Geometry: final body of the model. Coordinates: model frame, mm. A direction names the side the tool comes from. Round coordinates to 2 decimals unless told otherwise and drop trailing zeros. Loops run counter-clockwise (first coordinate to the right, second up) from the corner with the lowest first, then second, coordinate; pieces in that order, holes last. Notation, with made-up numbers: M 13.25,15.25 L 33.25,15.25 A18 ccw 33.25,29.25 Z; hole C 52,-18.5 d7. An arc over 180 degrees is marked long. Return JSON: item names as keys, results as strings.
Autodesk Fusion 360 part; units mm, degrees
sketch "Sketch1" plane through (0, 0, 0) normal (0, 0, 1) x (1, 0, 0) in component "Headpost"
  line L0 (7.5, -5) -> (-7.5, -5)
  line L1 (-7.5, -5) -> (-7.5, 5)
  line L2 (-7.5, 5) -> (7.5, 5)
  line L3 (7.5, 5) -> (7.5, -5)
  line L4 (7.5, -5) -> (-7.5, 5) construction
  line L5 (-7.5, -5) -> (7.5, 5) construction
  dimension "d1" = 15
  dimension "d2" = 10
extrude "Extrude1" add sketch "Sketch1" along normal blind 10 in component "Headpost"
sketch "Sketch2" plane through (0, 0, 10) normal (0, 0, 1) x (-1, 0, 0) in component "Headpost"
  line L0 (-7.5, -5) -> (7.5, -5)
  line L1 (7.5, -5) -> (7.5, 5)
  line L2 (7.5, 5) -> (-7.5, 5)
  line L3 (-7.5, 5) -> (-7.5, -5)
  line L4 (6, 3.5) -> (-6, 3.5)
  line L5 (-6, 3.5) -> (-6, -3.5)
  line L6 (-6, -3.5) -> (6, -3.5)
  line L7 (6, -3.5) -> (6, 3.5)
  dimension "d5" = -1.5
extrude "Extrude2" cut sketch "Sketch2" against normal blind 15 contours L4 L5 L6 L7 in component "Headpost"
sketch "Sketch3" plane through (-7.5, 0, 0) normal (-1, 0, 0) x (0, -1, 0) in component "Headpost"
  line L0 (-5, 0) -> (5, 0)
  line L1 (5, 0) -> (5, 10)
  line L2 (5, 10) -> (-5, 10)
  line L3 (-5, 10) -> (-5, 0)
  line L4 (-5, 10) -> (5, 10)
  line L5 (5, 10) -> (5, 8)
  line L6 (5, 8) -> (-5, 8)
  line L7 (-5, 8) -> (-5, 10)
  dimension "d8" = 10
  dimension "d9" = 2
extrude "Extrude3" add sketch "Sketch3" along normal blind 7.5 contours L1 L2 L3 L4 L5 L6 L7 in component "Headpost"
sketch "Sketch4" plane through (7.5, 0, 0) normal (1, 0, 0) x (0, 1, 0) in component "Headpost"
  line L0 (-5, 0) -> (5, 0)
  line L1 (5, 0) -> (5, 10)
  line L2 (5, 10) -> (-5, 10)
  line L3 (-5, 10) -> (-5, 0)
  line L4 (-5, 10) -> (5, 10)
  line L5 (5, 10) -> (5, 8)
  line L6 (5, 8) -> (-5, 8)
  line L7 (-5, 8) -> (-5, 10)
  dimension "d12" = 2
extrude "Extrude4" add sketch "Sketch4" along normal blind 7.5 contours L1 L2 L3 L4 L5 L6 L7 in component "Headpost"
fillet "Fillet1" radius 1.25 2 edges at (6, -3.5, 5) (6, 3.5, 5) in component "Headpost"
fillet "Fillet2" radius 1.25 2 edges at (-6, 3.5, 5) (-6, -3.5, 5) in component "Headpost"
fillet "Fillet3" radius 1.25 4 edges at (15, -5, 9) (15, 5, 9) (-15, 5, 9) (-15, -5, 9) in component "Headpost"
sketch "Sketch5" plane through (0, 0, 10) normal (0, 0, 1) x (-1, 0, 0) in component "Headpost"
  arc A0 (15, 3.75) -> (13.75, 5) centre (13.75, 3.75) ccw
  line L0 (13.75, 5) -> (-13.75, 5)
  arc A1 (-13.75, 5) -> (-15, 3.75) centre (-13.75, 3.75) ccw
  line L1 (-15, 3.75) -> (-15, -3.75)
  arc A2 (-15, -3.75) -> (-13.75, -5) centre (-13.75, -3.75) ccw
  line L2 (-13.75, -5) -> (13.75, -5)
  arc A3 (13.75, -5) -> (15, -3.75) centre (13.75, -3.75) ccw
  line L3 (15, -3.75) -> (15, 3.75)
  line L4 (-4.75, 3.5) -> (4.75, 3.5)
  arc A4 (6, 2.25) -> (4.75, 3.5) centre (4.75, 2.25) ccw
  line L5 (6, 2.25) -> (6, -2.25)
  arc A5 (4.75, -3.5) -> (6, -2.25) centre (4.75, -2.25) ccw
  line L6 (4.75, -3.5) -> (-4.75, -3.5)
  arc A6 (-6, -2.25) -> (-4.75, -3.5) centre (-4.75, -2.25) ccw
  line L7 (-6, -2.25) -> (-6, 2.25)
  arc A7 (-4.75, 3.5) -> (-6, 2.25) centre (-4.75, 2.25) ccw
  line L8 (13, -5) -> (9, -5)
  line L9 (9, -5) -> (9, 5)
  line L10 (9, 5) -> (13, 5)
  line L11 (13, 5) -> (13, -5)
  line L12 (-9, -5) -> (-13, -5)
  line L13 (-13, -5) -> (-13, 5)
  line L14 (-13, 5) -> (-9, 5)
  line L15 (-9, 5) -> (-9, -5)
  dimension "d21" = 4
  dimension "d22" = 10
  dimension "d23" = 3
  dimension "d24" = 4
  dimension "d25" = 10
  dimension "d26" = 3
extrude "Extrude5" add sketch "Sketch5" along normal blind 1 contours L0 L2 L8 L9 L10 L11 in component "Headpost"
sketch "Sketch6" plane through (0, 0, 10) normal (0, 0, 1) x (-1, 0, 0) in component "Headpost"
  line L0 (-4.75, 3.5) -> (4.75, 3.5)
  arc A0 (6, 2.25) -> (4.75, 3.5) centre (4.75, 2.25) ccw
  line L1 (6, 2.25) -> (6, -2.25)
  arc A1 (4.75, -3.5) -> (6, -2.25) centre (4.75, -2.25) ccw
  line L2 (4.75, -3.5) -> (-4.75, -3.5)
  arc A2 (-6, -2.25) -> (-4.75, -3.5) centre (-4.75, -2.25) ccw
  line L3 (-6, -2.25) -> (-6, 2.25)
  arc A3 (-4.75, 3.5) -> (-6, 2.25) centre (-4.75, 2.25) ccw
  line L4 (9, -5) -> (9, 5)
  line L5 (9, 5) -> (-13.75, 5)
  arc A4 (-13.75, 5) -> (-15, 3.75) centre (-13.75, 3.75) ccw
  line L6 (-15, 3.75) -> (-15, -3.75)
  arc A5 (-15, -3.75) -> (-13.75, -5) centre (-13.75, -3.75) ccw
  line L7 (-13.75, -5) -> (9, -5)
  line L8 (-9, -5) -> (-13, -5)
  line L9 (-13, -5) -> (-13, 5)
  line L10 (-13, 5) -> (-9, 5)
  line L11 (-9, 5) -> (-9, -5)
  dimension "d29" = 4
  dimension "d30" = 10
  dimension "d31" = 3
extrude "Extrude6" add sketch "Sketch6" along normal blind 1 contours L5 L7 L8 L9 L10 L11 in component "Headpost"
fillet "Fillet4" radius 0.5 2 edges at (-13, -5, 10.5) (-9, -5, 10.5) in component "Headpost"
fillet "Fillet5" radius 0.5 2 edges at (9, -5, 10.5) (13, -5, 10.5) in component "Headpost"
fillet "Fillet6" radius 0.5 2 edges at (13, 5, 10.5) (9, 5, 10.5) in component "Headpost"
fillet "Fillet7" radius 0.5 2 edges at (-9, 5, 10.5) (-13, 5, 10.5) in component "Headpost"
sketch "Sketch7" plane through (0, 5, 0) normal (0, 1, 0) x (-1, 0, 0) in component "Headpost"
  line L0 (13.75, 10) -> (12.5, 10)
  line L1 (12.5, 10) -> (12.5, 11)
  line L2 (12.5, 11) -> (9.5, 11)
  line L3 (9.5, 11) -> (9.5, 10)
  line L4 (9.5, 10) -> (-9.5, 10)
  line L5 (-9.5, 10) -> (-9.5, 11)
  line L6 (-9.5, 11) -> (-12.5, 11)
  line L7 (-12.5, 11) -> (-12.5, 10)
  line L8 (-12.5, 10) -> (-13.75, 10)
  line L9 (-13.75, 10) -> (-13.75, 8)
  line L10 (-13.75, 8) -> (-7.5, 8)
  line L11 (-7.5, 8) -> (-7.5, 0)
  line L12 (-7.5, 0) -> (7.5, 0)
  line L13 (7.5, 0) -> (7.5, 8)
  line L14 (7.5, 8) -> (13.75, 8)
  line L15 (13.75, 8) -> (13.75, 10)
  line L16 (-6, 3) -> (6, 3)
  line L17 (6, 3) -> (6, 1)
  line L18 (6, 1) -> (-6, 1)
  line L19 (-6, 1) -> (-6, 3)
  dimension "d42" = 2
extrude "Extrude7" cut sketch "Sketch7" against normal blind 3 contours L16 L17 L18 L19 in component "Headpost"
sketch "Sketch8" plane through (0, -5, 0) normal (0, -1, 0) x (1, 0, 0) in component "Headpost"
  line L0 (13.75, 10) -> (12.5, 10)
  line L1 (12.5, 10) -> (12.5, 11)
  line L2 (12.5, 11) -> (9.5, 11)
  line L3 (9.5, 11) -> (9.5, 10)
  line L4 (9.5, 10) -> (-9.5, 10)
  line L5 (-9.5, 10) -> (-9.5, 11)
  line L6 (-9.5, 11) -> (-12.5, 11)
  line L7 (-12.5, 11) -> (-12.5, 10)
  line L8 (-12.5, 10) -> (-13.75, 10)
  line L9 (-13.75, 10) -> (-13.75, 8)
  line L10 (-13.75, 8) -> (-7.5, 8)
  line L11 (-7.5, 8) -> (-7.5, 0)
  line L12 (-7.5, 0) -> (7.5, 0)
  line L13 (7.5, 0) -> (7.5, 8)
  line L14 (7.5, 8) -> (13.75, 8)
  line L15 (13.75, 8) -> (13.75, 10)
  line L16 (-6, 3) -> (6, 3)
  line L17 (6, 3) -> (6, 1)
  line L18 (6, 1) -> (-6, 1)
  line L19 (-6, 1) -> (-6, 3)
  dimension "d45" = 2
extrude "Extrude8" cut sketch "Sketch8" against normal blind 3 contours L16 L17 L18 L19 in component "Headpost"
sketch "Sketch11" plane through (0, 0, 8) normal (0, 0, -1) x (1, 0, 0) in component "Headpost"
  arc A0 (13.75, -5) -> (15, -3.75) centre (13.75, -3.75) ccw
  line L0 (15, -3.75) -> (15, 3.75)
  arc A1 (15, 3.75) -> (13.75, 5) centre (13.75, 3.75) ccw
  line L1 (13.75, 5) -> (7.5, 5)
  line L2 (7.5, 5) -> (7.5, -5)
  line L3 (7.5, -5) -> (13.75, -5)
  line L4 (-13, 5) -> (-9, 5)
  line L5 (-9, 5) -> (-9, -5)
  line L6 (-9, -5) -> (-13, -5)
  line L7 (-13, -5) -> (-13, 5)
  line L8 (-15, -3.75) -> (-15, 3.75)
  dimension "d48" = 4
  dimension "d49" = 10
  dimension "d50" = 2
extrude "Extrude9" cut sketch "Sketch11" against normal blind 1 contours L4 L5 L6 L7 in component "Headpost"
fillet "Fillet8" radius 0.5 4 edges at (-9, 5, 8.5) (-13, 5, 8.5) (-13, -5, 8.5) (-9, -5, 8.5) in component "Headpost"
sketch "Sketch12" plane through (0, 0, 8) normal (0, 0, -1) x (1, 0, 0) in component "Headpost"
  arc A0 (13.75, -5) -> (15, -3.75) centre (13.75, -3.75) ccw
  line L0 (15, -3.75) -> (15, 3.75)
  arc A1 (15, 3.75) -> (13.75, 5) centre (13.75, 3.75) ccw
  line L1 (13.75, 5) -> (7.5, 5)
  line L2 (7.5, 5) -> (7.5, -5)
  line L3 (7.5, -5) -> (13.75, -5)
  line L4 (9, 5) -> (13, 5)
  line L5 (13, 5) -> (13, -5)
  line L6 (13, -5) -> (9, -5)
  line L7 (9, -5) -> (9, 5)
  dimension "d55" = 4
  dimension "d56" = 10
  dimension "d57" = 2
extrude "Extrude10" cut sketch "Sketch12" against normal blind 1 contours L1 L3 L4 L5 L6 L7 in component "Headpost"
fillet "Fillet9" radius 0.5 4 edges at (13, 5, 8.5) (9, 5, 8.5) (9, -5, 8.5) (13, -5, 8.5) in component "Headpost"
sketch "Sketch9" plane through (0, 0, 0) normal (1, 0, 0) x (0, 1, 0) in component "Headpost"
component "Headpost" placed x (1, 0, 0) y (0, 1, 0) z (0, 0, 1) at (-0.1721, 0.3027, 0.1438)
Q1. Reachability of faces 1 (the flat face through (8.828, 0.4, 8.6)), 2 (the flat face through (8, 0, 8.144)), 3 (the flat face through (8.828, 0.2, 10.6)), 4 (the flat face through (-7.672, 0, 4)) from +Z, -Z, +X, -X, +Y, -Y: full face, straight path, thin tool, end or side. Return the list, or none.
Determined:
{"face 1": "-Z, +Y, -Y", "face 2": "-Z, +X, +Y, -Y", "face 3": "+Z, +Y, -Y", "face 4": "-Z, -X, +Y, -Y"}
Q2. Pull-direction query (X, two-part tool) for faces 5 (the flat face through (0, -4.697, 6)), 6 (the cylindrical face through (-14.816, -4.321, 9.158)), 7 (the flat face through (-0.1, 3.803, 0.7)); classes: pulls with the +X half, pulls with the -X half, needs draft (parallel to the pull), parting line crosses it, or undercut.
Determined:
{"face 5": "needs draft", "face 6": "pulls with the -X half", "face 7": "undercut"}
Q3. Section query C-C (z = 5.75). Output: boundary loops of the cut face in (x, y).
Determined:
{"outline": "M -7.67,-4.7 L 7.33,-4.7 L 7.33,5.3 L -7.67,5.3 Z; hole M -6.17,-1.95 A1.25 ccw -4.92,-3.2 L 4.58,-3.2 A1.25 ccw 5.83,-1.95 L 5.83,2.55 A1.25 ccw 4.58,3.8 L -4.92,3.8 A1.25 ccw -6.17,2.55 Z"}
Q4. Pin query (flat end, axial travel): pin 1 (2 mm diameter, centred on y = -2.5, z = 2.5, fed in from -X); pin 2 (1.4 mm diameter, centred on x = -1, y = -4, fed in from +Z); pin 3 (0.8 mm diameter, centred on y = -1.5, z = 10.5, fed in from -X); pin 4 (2 mm diameter, centred on x = 1.5, y = 1, fed in from -Z). Return the tip coordinate at first contact, or that it passes through.
Determined:
{"pin 1": "stops at x = -7.67", "pin 2": "stops at z = 10.14", "pin 3": "stops at x = -15.17", "pin 4": "passes through"}
Q5. Material intervals for L1, parallel to X at y = 0, z = 8.5; L2, parallel to Y at x = 0.25, z = 5.75; L3, parallel to X at y = 1.25, z = 1.5, sorted ascending.
Determined:
{"L1": "x = -15.17 to -13.17, -9.17 to -6.17, 5.83 to 8.83, 12.83 to 14.83", "L2": "y = -4.7 to -3.2, 3.8 to 5.3", "L3": "x = -7.67 to -6.17, 5.83 to 7.33"}
Q6. Section query A-A (z = 2.5). Output: boundary loops of the cut face in (x, y).
Determined:
{"outline": "M -7.67,-4.7 L -6.17,-4.7 L -6.17,5.3 L -7.67,5.3 Z; M 5.83,-4.7 L 7.33,-4.7 L 7.33,5.3 L 5.83,5.3 Z"}
Q7. Section query D-D (x = -5.5). Output: boundary loops of the cut face in (y, z).
Determined:
{"outline": "M -4.7,0.14 L -3.06,0.14 L -3.06,1.14 L -4.7,1.14 Z; M -4.7,3.14 L -3.06,3.14 L -3.06,10.14 L -4.7,10.14 Z; M 3.66,0.14 L 5.3,0.14 L 5.3,1.14 L 3.66,1.14 Z; M 3.66,3.14 L 5.3,3.14 L 5.3,10.14 L 3.66,10.14 Z"}
Q8. Section query B-B (x = 0.5). Output: boundary loops of the cut face in (y, z).
Determined:
{"outline": "M -4.7,0.14 L -3.2,0.14 L -3.2,1.14 L -4.7,1.14 Z; M -4.7,3.14 L -3.2,3.14 L -3.2,10.14 L -4.7,10.14 Z; M 3.8,0.14 L 5.3,0.14 L 5.3,1.14 L 3.8,1.14 Z; M 3.8,3.14 L 5.3,3.14 L 5.3,10.14 L 3.8,10.14 Z"}
